from build123d import *

# Parameters (mm, degrees)
BOSS_EXTRUDE1_DEPTH = 12.7
SKETCH2_R           = 1.5
CUT_EXTRUDE1_DEPTH  = 3.2
SKETCH3_R           = 2
BOSS_EXTRUDE2_DEPTH = 9.5


with BuildPart() as part:
    # Sketch1 → Boss-Extrude1 (new body)
    with BuildSketch(Plane(origin=(0, 0, 0), x_dir=(1, 0, 0), z_dir=(0, 1, 0))):
        Polygon((0, 6.350852961), (-5.5, 3.175426481), (-5.5, -3.175426481), (0, -6.350852961), (5.5, -3.175426481), (5.5, 3.175426481), align=None)
    extrude(amount=BOSS_EXTRUDE1_DEPTH)

    # Sketch2 → Cut-Extrude1 (cut)
    with BuildSketch(Plane(origin=(0, 12.7, 0), x_dir=(1, 0, 0), z_dir=(0, 1, 0))):
        with Locations(Location((0, 0, 0), (0, 0, 270))):
            Circle(SKETCH2_R)
    extrude(amount=-CUT_EXTRUDE1_DEPTH, mode=Mode.SUBTRACT)

    # Sketch3 → Boss-Extrude2 (add)
    with BuildSketch(Plane.XZ):
        with Locations(Location((0, 0, 0), (0, 0, 270))):
            Circle(SKETCH3_R)
    extrude(amount=BOSS_EXTRUDE2_DEPTH)


solid = part.part
Verification items for the finished model (mm, model axes). Round coordinates to 2 decimals unless told otherwise and drop trailing zeros. Loops run counter-clockwise (first coordinate to the right, second up) from the corner with the lowest first, then second, coordinate; pieces in that order, holes last. Notation, with made-up numbers: (13, 75) - (45, 75) arc R24 cw to (45, 89) - close; hole circle Ø4 at (-37, -39). An arc over 180 degrees is marked (long way). Use one line per item in the form item = value.
1. Section check C-C on x = -1. Record the cut outline in (y, z).
A:
outline = (-9.5, -1.73) - (0, -1.73) - (0, -5.77) - (12.7, -5.77) - (12.7, -1.12) - (9.5, -1.12) - (9.5, 1.12) - (12.7, 1.12) - (12.7, 5.77) - (0, 5.77) - (0, 1.73) - (-9.5, 1.73) - close
2. Draft check along X on faces 1 (the flat face through (0, 0, 3)), 2 (the flat face through (0, 9.5, 0)), 3 (the cylindrical face through (0.45, 11.12, 1.43)), 4 (the cylindrical face through (-2, -5, 0)). Enter one of: pulls with the +X half, pulls with the -X half, needs draft (parallel to the pull), parting line crosses it, or undercut.
A:
face_1 = needs draft
face_2 = undercut
face_3 = undercut
face_4 = parting line crosses it
3. Scan lines: probe 1 along X at (y, z) = (10.5, 0); probe 2 along Y at (x, z) = (0.75, -0.75); probe 3 along Y at (x, z) = (-2.5, -3.5). Record each from-to range of solid material in increasing order.
A:
probe_1 = -5.5 to -1.5, 1.5 to 5.5
probe_2 = -9.5 to 9.5
probe_3 = 0 to 12.7
4. Section check D-D on y = -6.25. Record the cut outline in (x, z), and give its area (3 significant figures).
A:
outline = circle Ø4 at (0, 0)
area = 12.6 mm²
5. Gauge pin test, flat ends, axial feed: pin 1 Ø3 at (x, y) = (-3.5, 7) entering from +Z; pin 2 Ø2.5 at (x, z) = (0, 0) entering from +Y; pin 3 Ø2 at (y, z) = (-1.5, -1) entering from +X. Record the tip position at first contact, or that the pin passes through.
A:
pin_1 = 5.2
pin_2 = 9.5
pin_3 = 2
6. Section check A-A on z = 0. Record the cut outline in (x, y).
A:
outline = (-5.5, 0) - (-2, 0) - (-2, -9.5) - (2, -9.5) - (2, 0) - (5.5, 0) - (5.5, 12.7) - (1.5, 12.7) - (1.5, 9.5) - (-1.5, 9.5) - (-1.5, 12.7) - (-5.5, 12.7) - close
7. Section check B-B on y = 10.5. Record the cut outline in (x, z), and give its area (3 significant figures).
A:
outline = (-5.5, -3.18) - (0, -6.35) - (5.5, -3.18) - (5.5, 3.18) - (0, 6.35) - (-5.5, 3.18) - close; hole circle Ø3 at (0, 0)
area = 97.7 mm²
